```python
from build123d import *

# Parameters (mm, degrees)
SKETCH_2_R               = 27.5
SKETCH_2_R_2             = 0.525
EXTRUDE_1_DEPTH          = 5
SKETCH_5_W               = 5
SKETCH_5_H               = 4
CUT_EXTRUDE_1_DEPTH      = 44.181327292
PATTERN_CIRCULAR_1_COUNT = 4
CUT_EXTRUDE_2_DEPTH      = 2
PATTERN_CIRCULAR_2_COUNT = 4
SKETCH_7_R               = 2.5
CUT_EXTRUDE_3_DEPTH      = 40.210967853
SKETCH_8_R               = 1
CUT_EXTRUDE_4_DEPTH      = 1
PATTERN_CIRCULAR_3_COUNT = 4


with BuildPart() as part:
    # Sketch 2 → Extrude 1 (new body)
    with BuildSketch(Plane(origin=(0, 0, 0), x_dir=(1, 0, 0), z_dir=(0, 1, 0))):
        with Locations(Location((0, 0, 0), (0, 0, 270))):
            Circle(SKETCH_2_R)
        with Locations(Location((0, 22.5, 0), (0, 0, 270))):
            Circle(SKETCH_2_R_2, mode=Mode.SUBTRACT)
        with Locations(Location((22.5, -2e-09, 0), (0, 0, 270))):
            Circle(SKETCH_2_R_2, mode=Mode.SUBTRACT)
        with Locations(Location((-2e-09, -22.500000002, 0), (0, 0, 270))):
            Circle(SKETCH_2_R_2, mode=Mode.SUBTRACT)
        with Locations(Location((-22.500000002, 0, 0), (0, 0, 270))):
            Circle(SKETCH_2_R_2, mode=Mode.SUBTRACT)
        Polygon((-13.788582233, 19.445436483), (13.788582233, 19.445436483), (0, 5.656854249), align=None, mode=Mode.SUBTRACT)
        Polygon((-19.445436483, 13.788582233), (-19.445436483, -13.788582233), (-5.656854249, 0), align=None, mode=Mode.SUBTRACT)
        Polygon((-13.788582233, -19.445436483), (13.788582233, -19.445436483), (0, -5.656854249), align=None, mode=Mode.SUBTRACT)
        Polygon((19.445436483, 13.788582233), (19.445436483, -13.788582233), (5.656854249, 0), align=None, mode=Mode.SUBTRACT)
    extrude(amount=EXTRUDE_1_DEPTH)

    # Sketch 5 → Cut-Extrude 1 (cut, through all)
    with BuildSketch(Plane(origin=(2.828427515, 4.42e-07, -2.828427515), x_dir=(0.7071067811865507, 0, 0.7071067811865444), z_dir=(-0.7071067811865401, -1.1050996923684133e-07, 0.7071067811865465))):
        with Locations((0, 2.5)):
            Rectangle(SKETCH_5_W, SKETCH_5_H)
    cut_extrude_1 = extrude(amount=-CUT_EXTRUDE_1_DEPTH, mode=Mode.SUBTRACT)

    # Pattern Circular 1: Cut-Extrude 1 ×4 about axis
    pattern_circular_1_axis = Axis((0, 0, 0), (0, 1, 0))
    for i in range(1, PATTERN_CIRCULAR_1_COUNT):
        add(cut_extrude_1.rotate(pattern_circular_1_axis, i * 360 / PATTERN_CIRCULAR_1_COUNT), mode=Mode.SUBTRACT)

    # Sketch 6 → Cut-Extrude 2 (cut)
    with BuildSketch(Plane(origin=(0, 5, 0), x_dir=(1, 0, 0), z_dir=(0, 1, 0))):
        Polygon((-1.226687162, 4.762221068), (-4.762221068, 1.226687162), (-7.590648193, 4.055114287), (-4.055114287, 7.590648193), align=None)
        Polygon((-10.419075318, 13.954609224), (-7.590648193, 11.126182099), (-11.126182099, 7.590648193), (-13.954609224, 10.419075318), align=None)
        Polygon((-13.0009557, 16.536489606), (-16.536489606, 13.0009557), (-19.364916731, 15.829382825), (-15.829382825, 19.364916731), align=None)
    cut_extrude_2 = extrude(amount=-CUT_EXTRUDE_2_DEPTH, mode=Mode.SUBTRACT)

    # Pattern Circular 2: Cut-Extrude 2 ×4 about axis
    pattern_circular_2_axis = Axis((0, 0, 0), (0, 1, 0))
    for i in range(1, PATTERN_CIRCULAR_2_COUNT):
        add(cut_extrude_2.rotate(pattern_circular_2_axis, i * 360 / PATTERN_CIRCULAR_2_COUNT), mode=Mode.SUBTRACT)

    # Sketch 7 → Cut-Extrude 3 (cut, through all)
    with BuildSketch(Plane(origin=(0, 5, 0), x_dir=(1, 0, 0), z_dir=(0, 1, 0))):
        with Locations(Location((0, 0, 0), (0, 0, 270))):
            Circle(SKETCH_7_R)
    extrude(amount=-CUT_EXTRUDE_3_DEPTH, mode=Mode.SUBTRACT)

    # Sketch 8 → Cut-Extrude 4 (cut)
    with BuildSketch(Plane(origin=(0, 5, 0), x_dir=(1, 0, 0), z_dir=(0, 1, 0))):
        with Locations(Location((-22.500000002, 0, 0), (0, 0, 270))):
            Circle(SKETCH_8_R)
    cut_extrude_4 = extrude(amount=-CUT_EXTRUDE_4_DEPTH, mode=Mode.SUBTRACT)

    # Pattern Circular 3: Cut-Extrude 4 ×4 about axis
    pattern_circular_3_axis = Axis((0, 0, 0), (0, 1, 0))
    for i in range(1, PATTERN_CIRCULAR_3_COUNT):
        add(cut_extrude_4.rotate(pattern_circular_3_axis, i * 360 / PATTERN_CIRCULAR_3_COUNT), mode=Mode.SUBTRACT)


solid = part.part
```
For this review, take the finished solid that the model builds, in its own axes (mm). A direction names the side the tool comes from. Give positions to 0.01 mm unless a question says otherwise; leave off trailing zeros. Write each loop counter-clockwise with the first axis right and the second up, starting at its lowest first coordinate (ties: lowest second). Pieces come first, ordered by that corner, then holes.
Item 1: Insertion check: P1, Ø2, axis at y = 4.5, z = 12, coming from the +X side; P2, Ø0.6, axis at x = -22.5, z = 0.5, coming from the +Y side; P3, Ø1.5, axis at x = 6.5, y = 2.5, coming from the +Z side. Each pin has a flat end and moves straight along its axis. Give the tip position at first contact, or say it passes through.
Item 2: Take a section at B-B (z = -12). Give the boundary of the cut face in (x, y), and give its area (3 significant figures).
Item 3: Take a section at A-A (y = 1.2). Give the number of separate pieces and of enclosed holes in the cut face, and give its area (3 significant figures).
Item 4: Wall thickness on probe 1 along Z at (x, y) = (16, 2.1); probe 2 along X at (y, z) = (3.9, -12.5); probe 3 along X at (y, z) = (1.7, -7.5): over which ranges is each line inside the solid? List them lowest first.
Item 5: Machinability: for faces 1 (the face through (9.213, 2.719, -12.749)), 2 (the face through (-0.7, 4, -22.5)), 3 (the face through (6.991, 2.465, -12.648)), which of the approach directions +Z, -Z, +X, -X, +Y, -Y give a long, thin tool a straight path to every point of the face, cutting with its end or side? Answer none if there is none.
Established:
1. P1: stops at x = 25.2
1. P2: stops at y = 4
1. P3: stops at z = 26.89
2. outline: (-24.74, 0) - (-19.45, 0) - (-19.45, 5) - (-24.74, 5) - close; (-17.66, 0) - (-6.34, 0) - (-6.34, 5) - (-8.46, 5) - (-8.46, 0.5) - (-15.54, 0.5) - (-15.54, 4.5) - (-12.37, 4.5) - (-12.37, 5) - (-17.66, 5) - close; (6.34, 0) - (17.66, 0) - (17.66, 5) - (12.37, 5) - (12.37, 4.5) - (15.54, 4.5) - (15.54, 0.5) - (8.46, 0.5) - (8.46, 5) - (6.34, 5) - close; (19.45, 0) - (24.74, 0) - (24.74, 5) - (19.45, 5) - close
2. area: 106 mm2
3. separate pieces: 1
3. enclosed holes: 9
3. area: 1,120 mm2
4. probe 1: z = -22.37 to -19.54, -12.46 to -10.34, 10.34 to 12.46, 19.54 to 22.37
4. probe 2: x = -24.49 to -19.45, -18.16 to -16.04, -8.96 to -6.84, 6.84 to 8.96, 16.04 to 18.16, 19.45 to 24.49
4. probe 3: x = -26.46 to -19.45, -13.16 to -11.04, -3.96 to -1.84, 1.84 to 3.96, 11.04 to 13.16, 19.45 to 26.46
5. face 1: none
5. face 2: +Y
5. face 3: +Y, -Y
